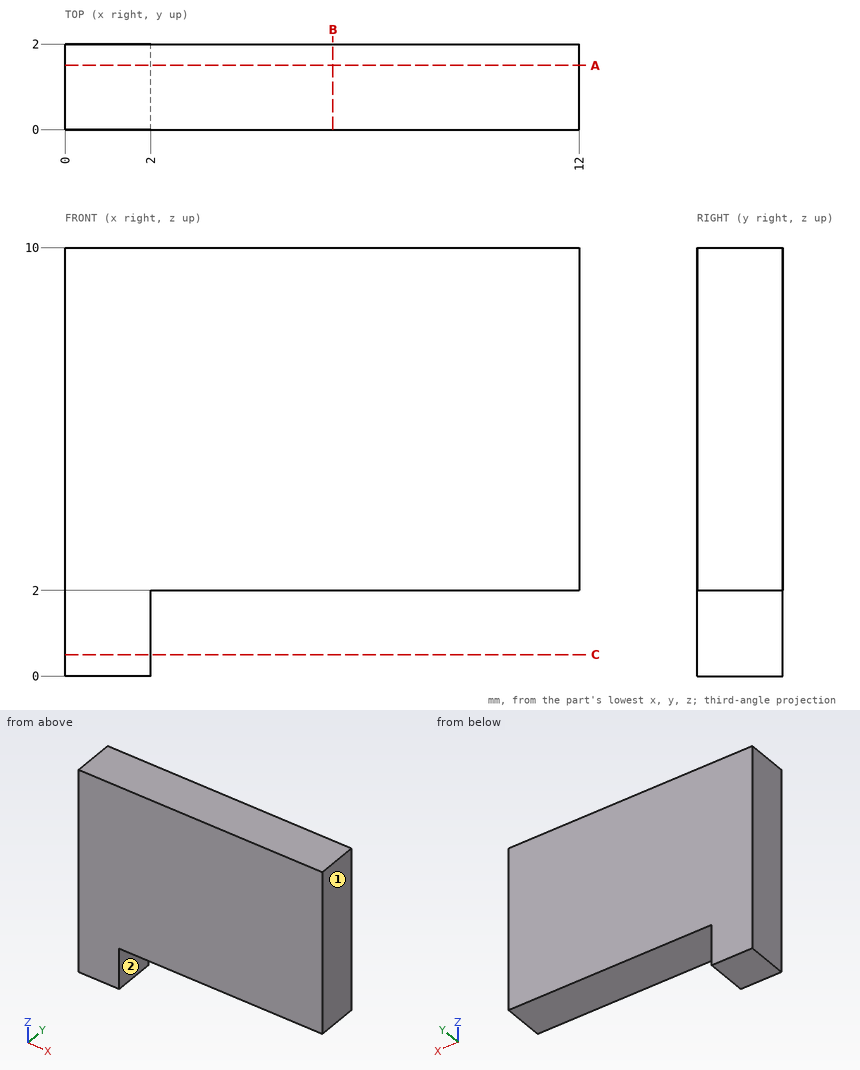
Input: dimensioned drawing with shaded views. Units: mm. Origin: part minimum x, y, z. A direction names the side the tool comes from. Round coordinates to 2 decimals unless told otherwise and drop trailing zeros. Order: outer loops, then holes, each group sorted by start corner. A loop starts at its lowest first (then second) coordinate and runs counter-clockwise, first axis right, second up. Notation, with made-up numbers: (16.25, 15.5) -> (75.25, 15.5) arc R22 cw to (75.25, 43.5) -> close; hole circle Ø7 at (-34, 43). An arc over 180 degrees is marked (long way). Put each result on its own line as item: value. Start each with the question number.
Q1. Line query: probe 1 along Z at (x, y) = (3.75, 0.45); probe 2 along X at (y, z) = (1.55, 0.75). Output: solid intervals per line, ascending.
Q2. First-contact query: pin 1 (1.5 mm diameter, centred on x = 7.5, z = 8.5, fed in from -Y). Flat tip, straight axial feed; report the tip coordinate or a pass-through.
Q3. Section A-A on y = 1.5. Return the cut outline in (x, z).
Q4. Reachability of the marked faces 1 and 2 from +Z, -Z, +X, -X, +Y, -Y: full face, straight path, thin tool, end or side. Return the list, or none.
Q5. Section C-C on z = 0.5. Return the cut outline in (x, y).
Q6. Section B-B on x = 6.25. Return the cut outline in (y, z).
Ans:
1. probe 1: z = 2 to 10
1. probe 2: x = 0 to 2
2. pin 1: stops at y = 0
3. outline: (0, 0) -> (2, 0) -> (2, 2) -> (12, 2) -> (12, 10) -> (0, 10) -> close
4. face 1: +Z, -Z, +X, +Y, -Y
4. face 2: -Z, +X, +Y, -Y
5. outline: (0, 0) -> (2, 0) -> (2, 2) -> (0, 2) -> close
6. outline: (0, 2) -> (2, 2) -> (2, 10) -> (0, 10) -> close
